Geometry: final body of the model. Coordinates: model frame, mm. A direction names the side the tool comes from. Round coordinates to 2 decimals unless told otherwise and drop trailing zeros. Order: outer loops, then holes, each group sorted by start corner. A loop starts at its lowest first (then second) coordinate and runs counter-clockwise, first axis right, second up. Notation, with made-up numbers: (51.25, 43) - (100.25, 43) arc R12 cw to (100.25, 55) - close; hole circle Ø8 at (14, 73). An arc over 180 degrees is marked (long way). Put each result on its own line as item: value. Start each with the question number.
(1) Section A-A (y = 24.5). Output: boundary loops of the cut face in (x, z).
(2) Material intervals for L1, parallel to Z at x = 7, y = 38.5; L2, parallel to Z at x = 4, y = 7; L3, parallel to Z at x = 6.5, y = 12.5, sorted ascending. Write a range as [from, to].
(3) Pull-direction query (X, two-part tool) for faces 3 (the face through (4.669, 11.696, -60.954)), 4 (the face through (6.028, 41.114, -56.188)); classes: released by +X, released by -X, zero draft, split by the parting line, or undercut.
(4) Access query for faces 1 (the face through (6.028, 22.314, -56.148)), 2 (the face through (4, 3.214, -50)). Directions: +Z, -Z, +X, -X, +Y, -Y. A direction counts if a zero-diameter tool reaches every point of the face in a straight line with its end or side. Return the directions, or none.
(5) Pin query (flat end, axial travel): P1, Ø4, axis at x = 3, z = -48.5, coming from the +Y side; P2, Ø1.6, axis at x = 6.5, y = 39, coming from the +Z side; P3, Ø5, axis at y = 34.5, z = -59, coming from the -X side; P4, Ø1.2, axis at y = 17.71, z = -42.92, coming from the -X side. Return the tip coordinate at first contact, or that it passes through.
(6) Section B-B (x = 4.5). Count the separate pieces of the cut face and the enclosed holes in it, and give its area (3 significant figures).
(7) Section C-C (z = -56.5). Output: boundary loops of the cut face in (x, y).
Autodesk Inventor part; units mm, degrees
ref_plane "YZ Plane" through (0, 0, 0) normal (1, 0, 0) x (0, 1, 0)
ref_plane "XZ Plane" through (0, 0, 0) normal (0, 1, 0) x (-1, 0, 0)
ref_plane "XY Plane" through (0, 0, 0) normal (0, 0, 1) x (1, 0, 0)
sketch "Sketch1" plane through (0, 0, 0) normal (1, 0, 0) x (0, 1, 0)
  line L0 (3.2139, -35.6679) -> (20.2139, -35.6679)
  line L1 (20.2139, -35.6679) -> (20.2139, -63.6679)
  line L2 (20.2139, -63.6679) -> (3.2139, -63.6679)
  line L3 (3.2139, -63.6679) -> (3.2139, -35.6679)
  point P0 (0, 0)
  dimension "d0" = 17
  dimension "d1" = 28
extrude "Extrusion1" add sketch "Sketch1" along normal blind 8
sketch "Sketch2" plane through (8, 0, 0) normal (1, 0, 0) x (0, 0, -1)
  line L0 (63.6679, 3.2139) -> (63.6679, 20.2139)
  line L1 (63.6679, 20.2139) -> (53.6679, 20.2139)
  line L2 (53.6679, 20.2139) -> (53.6679, 42.2139)
  line L3 (53.6679, 42.2139) -> (63.6679, 42.2139)
  line L4 (63.6679, 42.2139) -> (63.6679, 20.2139)
  point P0 (0, 0)
  dimension "d4" = 10
  dimension "d5" = 22
extrude "Extrusion2" add sketch "Sketch2" against normal up to surface (8 mm away)
sketch "Sketch3" plane through (8, 20.2139, -53.6679) normal (0, 0, 1) x (1, 0, 0)
  line L0 (-8, 0) -> (0, 0)
  line L1 (-8, -17) -> (-8, 22)
  line L2 (-4, 0) -> (-8, 0)
  line L3 (-8, 0) -> (-8, 22)
  line L4 (-8, 22) -> (-4, 22)
  line L5 (-4, 22) -> (-4, 0)
  point P0 (-8, -20.2139)
  dimension "d8" = 4
extrude "Extrusion3" cut sketch "Sketch3" against normal through all
sketch "Sketch4" plane through (8, 0, 0) normal (1, 0, 0) x (0, 0, -1)
  circle A0 centre (42.9179, 5.7139) radius 1
  circle A1 centre (42.9179, 17.7139) radius 1
  circle A2 centre (50.9179, 5.7139) radius 1
  circle A3 centre (50.9179, 17.7139) radius 1
  line L0 (35.6679, 3.2139) -> (63.6679, 3.2139)
  line L1 (53.6679, 20.2139) -> (35.6679, 20.2139)
  line L2 (35.6679, 20.2139) -> (35.6679, 3.2139)
  point P0 (0, 0)
  dimension "d11" = 2
  dimension "d13" = 2
  dimension "d14" = 2
  dimension "d15" = 2
  dimension "d16" = 2.5
  dimension "d17" = 2.5
  dimension "d18" = 2.5
  dimension "d19" = 2.5
  dimension "d20" = 7.25
  dimension "d21" = 7.25
  dimension "d22" = 8
  dimension "d23" = 8
extrude "Extrusion4" cut sketch "Sketch4" against normal through all
sketch "Sketch5" plane through (0, 3.2139, -63.6679) normal (0, -1, 0) x (1, 0, 0)
  line L0 (4, 10) -> (4, 0)
  circle A0 centre (4, 4) radius 1.45
  circle A1 centre (4, 17) radius 1.45
  line L1 (8, 28) -> (8, 0)
  line L2 (0, 0) -> (8, 0)
  point P0 (0, 63.6679)
  dimension "d26" = 2.9
  dimension "d27" = 2.9
  dimension "d28" = 4
  dimension "d29" = 4
  dimension "d30" = 17
extrude "Extrusion5" cut sketch "Sketch5" against normal up to surface (17 mm away)
chamfer "Chamfer1" distance 0.2 angle 45 2 edges at (2.55, 3.2139, -46.6679) (2.55, 3.2139, -59.6679)
sketch "Sketch8" plane through (8, 0, 0) normal (1, 0, 0) x (0, 0, -1)
  circle A0 centre (40.6679, 11.7139) radius 1.45
  circle A1 centre (58.6679, 11.7139) radius 1.45
  circle A2 centre (49.6679, 11.7139) radius 1.45
  line L0 (53.6679, 20.2139) -> (35.6679, 20.2139)
  line L1 (35.6679, 3.2139) -> (63.6679, 3.2139)
  line L2 (63.6679, 3.2139) -> (63.6679, 42.2139)
  line L3 (35.6679, 20.2139) -> (35.6679, 3.2139)
  point P0 (0, 0)
  dimension "d53" = 8.5
  dimension "d54" = 8.5
  dimension "d55" = 8.5
  dimension "d56" = 2.9
  dimension "d57" = 2.9
  dimension "d58" = 2.9
  dimension "d59" = 5
  dimension "d60" = 14
  dimension "d61" = 5
extrude "Extrusion7" cut sketch "Sketch8" against normal through all
chamfer "Chamfer3" distance 1.4 angle 45 4 edges at (8, 5.7139, -41.9179) (8, 17.7139, -41.9179) (8, 17.7139, -49.9179) (8, 5.7139, -49.9179)
sketch "Sketch9" plane through (8, 0, 0) normal (1, 0, 0) x (0, 0, -1)
  circle A0 centre (56.1679, 25.2139) radius 0.9
  circle A1 centre (61.1679, 25.2139) radius 0.9
  circle A2 centre (61.1679, 40.2139) radius 0.9
  circle A3 centre (56.1679, 40.2139) radius 0.9
  line L0 (53.6679, 42.2139) -> (53.6679, 20.2139)
  line L1 (63.6679, 42.2139) -> (53.6679, 42.2139)
  line L2 (63.6679, 3.2139) -> (63.6679, 42.2139)
  line L3 (55.2679, 25.2139) -> (57.0679, 25.2139)
  line L4 (57.0679, 25.2139) -> (57.0679, 23.2139)
  line L5 (57.0679, 23.2139) -> (55.2679, 23.2139)
  line L6 (55.2679, 23.2139) -> (55.2679, 25.2139)
  line L7 (60.2679, 25.2139) -> (62.0679, 25.2139)
  line L8 (62.0679, 25.2139) -> (62.0679, 23.2139)
  line L9 (62.0679, 23.2139) -> (60.2679, 23.2139)
  line L10 (60.2679, 23.2139) -> (60.2679, 25.2139)
  line L11 (57.0679, 40.2139) -> (55.2679, 40.2139)
  line L12 (55.2679, 40.2139) -> (55.2679, 38.2139)
  line L13 (55.2679, 38.2139) -> (57.0679, 38.2139)
  line L14 (57.0679, 38.2139) -> (57.0679, 40.2139)
  line L15 (62.0679, 40.2139) -> (60.2679, 40.2139)
  line L16 (60.2679, 40.2139) -> (60.2679, 38.2139)
  line L17 (60.2679, 38.2139) -> (62.0679, 38.2139)
  line L18 (62.0679, 38.2139) -> (62.0679, 40.2139)
  arc A4 (55.2679, 23.2139) -> (57.0679, 23.2139) centre (56.1679, 23.2139) ccw
  arc A5 (60.2679, 23.2139) -> (62.0679, 23.2139) centre (61.1679, 23.1946) ccw
  arc A6 (60.2679, 38.2139) -> (62.0679, 38.2139) centre (61.1679, 38.2139) ccw
  arc A7 (55.2679, 38.2139) -> (57.0679, 38.2139) centre (56.1679, 38.2139) ccw
  point P0 (0, 0)
  dimension "d70" = 1.8
  dimension "d71" = 1.8
  dimension "d72" = 1.8
  dimension "d73" = 1.8
  dimension "d74" = 2.5
  dimension "d75" = 2
  dimension "d76" = 2
  dimension "d77" = 2.5
  dimension "d78" = 2.5
  dimension "d79" = 2.5
  dimension "d80" = 15
  dimension "d81" = 15
  dimension "d82" = 1.8
  dimension "d83" = 1.8
  dimension "d84" = 1.8
  dimension "d85" = 2
  dimension "d86" = 2
  dimension "d87" = 2
  dimension "d88" = 0.9
  dimension "d89" = 0.9
extrude "Extrusion8" cut sketch "Sketch9" against normal through all
properties part number "Z_probe_holder"
Checks:
1. outline: (4, -63.67) - (8, -63.67) - (8, -62.07) - (4, -62.07) - close; (4, -60.27) - (8, -60.27) - (8, -57.07) - (4, -57.07) - close; (4, -55.27) - (8, -55.27) - (8, -53.67) - (4, -53.67) - close
2. L1: z = [-63.67, -62.07], [-60.27, -57.07], [-55.27, -53.67]
2. L2: z = [-63.67, -61.12], [-58.22, -48.12], [-45.22, -35.67]
2. L3: z = [-63.67, -59.89], [-57.45, -50.89], [-48.45, -41.89], [-39.45, -35.67]
3. face 3: undercut
3. face 4: zero draft
4. face 1: +X, -X
4. face 2: +Z, -Z, +X, -X, -Y
5. P1: stops at y = 20.21
5. P2: stops at z = -53.67
5. P3: stops at x = 4
5. P4: passes through
6. separate pieces: 2
6. enclosed holes: 10
6. area: 551 mm²
7. outline: (0, 3.21) - (8, 3.21) - (8, 22.38) - (4, 22.38) - (4, 20.21) - (0, 20.21) - close; (4, 26.05) - (8, 26.05) - (8, 37.38) - (4, 37.38) - close; (4, 41.05) - (8, 41.05) - (8, 42.21) - (4, 42.21) - close
